The model under review builds one solid part; all positions refer to its coordinate system, in mm. Coordinates: 2 decimals unless noted, no trailing zeros. Order: outer loops, then holes, each group sorted by start corner. A loop starts at its lowest first (then second) coordinate and runs counter-clockwise, first axis right, second up. Notation, with made-up numbers: M -38.75,80.5 L -7.75,80.5 A28 cw -7.75,103.5 Z; hole C -35,-17.5 d7. An arc over 180 degrees is marked long. Write each question's results on one line, items separated by ' | '.
from build123d import *

# Parameters (mm, degrees)
BOSS_EXTRUDE1_DEPTH = 6.720839839
SKETCH2_W           = 80
SKETCH2_H           = 365
CUT_EXTRUDE1_DEPTH  = 517.04400614
FILLET1_R           = 5


with BuildPart() as part:
    # Sketch1 → Boss-Extrude1 (new body)
    with BuildSketch(Plane(origin=(0, 0, 0), x_dir=(-1.0, 0, 1.2419204428734467e-09), z_dir=(-1.2419204428734467e-09, 1.2419185922687681e-09, -1.0))):
        Polygon((372.500002384, 200.349256396), (373.839735985, 205.349251628), (377.499997616, 209.009498358), (382.499992847, 210.34924686), (402.500003576, 210.34924686), (407.499998808, 211.688995361), (411.160260439, 215.349256992), (412.49999404, 220.349252224), (412.49999404, 289.999991655), (392.500013113, 310.000002384), (-292.499989271, 310.000002384), (-412.49999404, 189.999997616), (-412.49999404, -189.999997616), (-292.499989271, -310.000002384), (392.500013113, -310.000002384), (412.49999404, -289.999991655), (412.49999404, 68.113133311), (411.160260439, 73.113135993), (407.499998808, 76.773390174), (402.500003576, 78.113131225), (382.499992847, 78.113131225), (377.499997616, 79.452879727), (373.839735985, 83.113133907), (372.500002384, 88.11313659), align=None)
    extrude(amount=-BOSS_EXTRUDE1_DEPTH)

    # Sketch2 → Cut-Extrude1 (cut, through all)
    with BuildSketch(Plane(origin=(0, 0, 0), x_dir=(-1.0, 0, 1.2419204428734473e-09), z_dir=(-1.2419204428734473e-09, 1.241918592268768e-09, -1.0))):
        with Locations((16.89999404, 0)):
            Rectangle(SKETCH2_W, SKETCH2_H)
    extrude(amount=-CUT_EXTRUDE1_DEPTH, mode=Mode.SUBTRACT)

    # Fillet1
    fillet1_edges = [part.edges().sort_by_distance(p)[0] for p in [
        (23.100005965, -182.500000004, 3.360419664),
        (23.100005965, 182.499999996, 3.360420117),
        (-56.899994035, 182.499999996, 3.360420217),
        (-56.899994035, -182.500000004, 3.360419763),
    ]]
    fillet(fillet1_edges, radius=FILLET1_R)


solid = part.part
1) Take a section at B-B on y = 127.5. State the section outline as (x, z) points.
Solutions:
outline: M -372.5,0 L -56.9,0 L -56.9,6.72 L -372.5,6.72 Z; M 23.1,0 L 412.5,0 L 412.5,6.72 L 23.1,6.72 Z
2) Take a section at A-A on x = -1.5. State the section outline as (y, z) points.
Solutions:
outline: M -310,0 L -182.5,0 L -182.5,6.72 L -310,6.72 Z; M 182.5,0 L 310,0 L 310,6.72 L 182.5,6.72 Z
3) To check wall thickness, follow line 1 along Y through (x, z) = (-2.5, 4.5); line 2 along X through (y, z) = (64.5, 4.75); line 3 along X through (y, z) = (98, 3.5). State the ranges of each line that lie inside material, in increasing order.
Solutions:
line 1: -310 to -182.5, 182.5 to 310 | line 2: -412.5 to -56.9, 23.1 to 412.5 | line 3: -372.5 to -56.9, 23.1 to 412.5
4) For pin 1 (2 mm diameter, centred on x = -397.5, z = 2.5, fed in from +Y); pin 2 (2 mm diameter, centred on y = 75.5, z = 4, fed in from -X); pin 3 (2 mm diameter, centred on y = 152.5, z = 5, fed in from -X), all flat-tipped, find the tip position at first contact; note any pin that passes through.
Solutions:
pin 1: y = 306 | pin 2: x = -409.77 | pin 3: x = -372.5
5) Take a section at D-D on y = -241. State the section outline as (x, z) points, plus the area to 3 significant figures.
Solutions:
outline: M -412.5,0 L 361.5,0 L 361.5,6.72 L -412.5,6.72 Z | area: 5,200 mm2
